from build123d import *

# Parameters (mm, degrees)
SKETCH1_W           = 25.4
SKETCH1_H           = 38.1
SKETCH1_R           = 2.0828
BOSS_EXTRUDE1_DEPTH = 6.35
SKETCH2_R           = 0.635
CUT_EXTRUDE1_DEPTH  = 3.556


with BuildPart() as part:
    # Sketch1 → Boss-Extrude1 (new body)
    with BuildSketch(Plane.XY):
        with Locations((12.7, 31.75)):
            Rectangle(SKETCH1_W, SKETCH1_H)
        with Locations((6.35, 19.05)):
            Circle(SKETCH1_R, mode=Mode.SUBTRACT)
        with Locations((6.35, 38.1)):
            Circle(SKETCH1_R, mode=Mode.SUBTRACT)
        with Locations((12.7, 44.45)):
            Circle(SKETCH1_R, mode=Mode.SUBTRACT)
        with Locations(Location((19.05, 19.05, 0), (0, 0, 180))):
            Circle(SKETCH1_R, mode=Mode.SUBTRACT)
        with Locations(Location((19.05, 38.1, 0), (0, 0, 180))):
            Circle(SKETCH1_R, mode=Mode.SUBTRACT)
    extrude(amount=BOSS_EXTRUDE1_DEPTH)

    # Sketch2 → Cut-Extrude1 (cut)
    with BuildSketch(Plane.XZ.offset(-12.7)):
        with Locations(Location((5.334, 3.175, 0), (0, 0, 270))):
            Circle(SKETCH2_R)
        with Locations(Location((20.066, 3.175, 0), (0, 0, 90))):
            Circle(SKETCH2_R)
    extrude(amount=-CUT_EXTRUDE1_DEPTH, mode=Mode.SUBTRACT)


solid = part.part
Work out the finished part from the listing and answer in its coordinate system (mm). A direction names the side the tool comes from. Give positions to 0.01 mm unless a question says otherwise; leave off trailing zeros. Order: outer loops, then holes, each group sorted by start corner. A loop starts at its lowest first (then second) coordinate and runs counter-clockwise, first axis right, second up. Notation, with made-up numbers: (-13, 63) -> (1, 63) arc R31 ccw to (1, 100) -> close; hole circle Ø8 at (19, 70). An arc over 180 degrees is marked (long way). One line per item, written item: value.
Item 1: A flat-ended cylindrical pin translates along its axis: P1, Ø0.8, axis at x = 5.334, z = 3.175, coming from the -Y side. Find the tip coordinate at first contact, or state that the pin passes through.
Answer sheet:
P1: y = 16.26
Item 2: Straight lines are drawn through the part: probe 1 along Y at (x, z) = (6.35, 3.25); probe 2 along Y at (x, z) = (7, 5.5); probe 3 along X at (y, z) = (44.5, 3). For each, find the intervals that lie inside material, in ascending order.
Answer sheet:
probe 1: 12.7 to 16.97, 21.13 to 36.02, 40.18 to 50.8
probe 2: 12.7 to 17.07, 21.03 to 36.12, 40.08 to 50.8
probe 3: 0 to 10.62, 14.78 to 25.4
Item 3: Determine the mould class of faces 3 (the cylindrical face through (19.436, 14.453, 3.092)), 4 (the flat face through (25.4, 31, 3)), 5 (the flat face through (13, 32, 0)) for opening direction X: released by +X, released by -X, zero draft, split by the parting line, or undercut.
Answer sheet:
face 3: undercut
face 4: released by +X
face 5: zero draft
Item 4: Find section D-D, the plane z = 2. Give the vertices of the cut face in (x, y), plus the area to 3 significant figures.
Answer sheet:
outline: (0, 12.7) -> (25.4, 12.7) -> (25.4, 50.8) -> (0, 50.8) -> close; hole circle Ø4.17 at (6.35, 19.05); hole circle Ø4.17 at (6.35, 38.1); hole circle Ø4.17 at (12.7, 44.45); hole circle Ø4.17 at (19.05, 19.05); hole circle Ø4.17 at (19.05, 38.1)
area: 900 mm²
Item 5: Find section C-C, the plane y = 19.05. Give the vertices of the cut face in (x, z), plus the area to 3 significant figures.
Answer sheet:
outline: (0, 0) -> (4.27, 0) -> (4.27, 6.35) -> (0, 6.35) -> close; (8.43, 0) -> (16.97, 0) -> (16.97, 6.35) -> (8.43, 6.35) -> close; (21.13, 0) -> (25.4, 0) -> (25.4, 6.35) -> (21.13, 6.35) -> close
area: 108 mm²
Item 6: Find section B-B, the plane y = 44.45. Give the vertices of the cut face in (x, z), plus the area to 3 significant figures.
Answer sheet:
outline: (0, 0) -> (10.62, 0) -> (10.62, 6.35) -> (0, 6.35) -> close; (14.78, 0) -> (25.4, 0) -> (25.4, 6.35) -> (14.78, 6.35) -> close
area: 135 mm²
Item 7: Find section A-A, the plane x = 6.35. Give the vertices of the cut face in (y, z), plus the area to 3 significant figures.
Answer sheet:
outline: (12.7, 0) -> (16.97, 0) -> (16.97, 6.35) -> (12.7, 6.35) -> close; (21.13, 0) -> (36.02, 0) -> (36.02, 6.35) -> (21.13, 6.35) -> close; (40.18, 0) -> (50.8, 0) -> (50.8, 6.35) -> (40.18, 6.35) -> close
area: 189 mm²
Item 8: A tool of negligible diameter and unlimited length cuts with its end or side. For faces 1 (the flat face through (0, 31, 3)), 2 (the cylindrical face through (5.763, 14.453, 3.643)), from which of +Z, -Z, +X, -X, +Y, -Y can it reach the whole face along a straight path? Write none if from no direction.
Answer sheet:
face 1: +Z, -Z, -X, +Y, -Y
face 2: -Y
